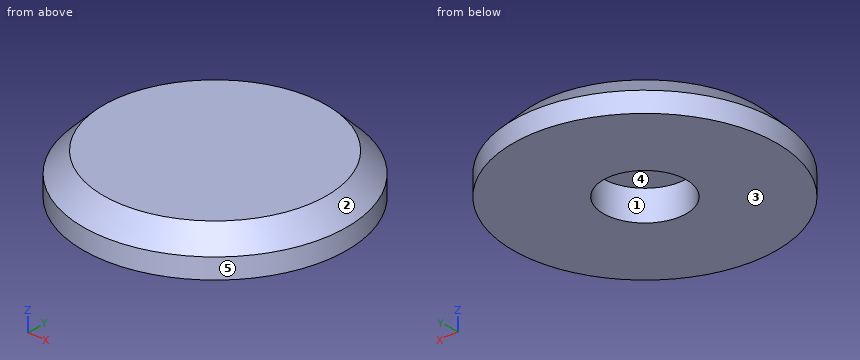
```python
from build123d import *

# Parameters (mm, degrees)
SKETCH1_R           = 3.7
BOSS_EXTRUDE1_DEPTH = 10
SKETCH2_R           = 5
BOSS_EXTRUDE2_DEPTH = 2
SKETCH3_R           = 13
SKETCH3_R_2         = 4.1
BOSS_EXTRUDE3_DEPTH = 4
SKETCH4_R           = 21.887313971
CUT_EXTRUDE1_DEPTH  = 23
CHAMFER2_SIZE       = 2
SKETCH5_R           = 5.500381587
BOSS_EXTRUDE4_DEPTH = 1


with BuildPart() as part:
    # Sketch1 → Boss-Extrude1 (new body)
    with BuildSketch(Plane.XY):
        Circle(SKETCH1_R)
    extrude(amount=BOSS_EXTRUDE1_DEPTH)

    # Sketch2 → Boss-Extrude2 (add)
    with BuildSketch(Plane(origin=(0, 0, 0), x_dir=(-1, 0, 0), z_dir=(0, 0, -1))):
        Circle(SKETCH2_R)
    extrude(amount=BOSS_EXTRUDE2_DEPTH)

    # Sketch4 → Cut-Extrude1 (cut)
    with BuildSketch(Plane(origin=(0, 0, 10), x_dir=(-1, 0, 0), z_dir=(0, 0, -1))):
        with Locations((0, 0.481738505)):
            Circle(SKETCH4_R)
    extrude(amount=CUT_EXTRUDE1_DEPTH, mode=Mode.SUBTRACT)


with BuildPart() as body_2:
    # Sketch3 → Boss-Extrude3 (new body)
    with BuildSketch(Plane.XY.offset(10)):
        Circle(SKETCH3_R)
        Circle(SKETCH3_R_2, mode=Mode.SUBTRACT)
    extrude(amount=BOSS_EXTRUDE3_DEPTH)

    # Chamfer2
    chamfer2_edges = [body_2.edges().sort_by_distance(p)[0] for p in [
        (-13, 0, 14),
    ]]
    chamfer(chamfer2_edges, length=CHAMFER2_SIZE)

    # Sketch5 → Boss-Extrude4 (add)
    with BuildSketch(Plane.XY.offset(14)):
        Circle(SKETCH5_R)
    extrude(amount=-BOSS_EXTRUDE4_DEPTH)


solid = body_2.part
```
Input: part model. Units: mm. Frame: model coordinates. Face numbers are marked on the shaded views. A direction names the side the tool comes from. Give positions to 0.01 mm unless a question says otherwise; leave off trailing zeros. Write each loop counter-clockwise with the first axis right and the second up, starting at its lowest first coordinate (ties: lowest second). Pieces come first, ordered by that corner, then holes. Notation, with made-up numbers: (-7.75, 19) - (49.25, 19) arc R23 ccw to (49.25, 39) - close; hole circle Ø2 at (82.5, -34.5). An arc over 180 degrees is marked (long way). Write item = value, one per line. Start each with the question number.
1. Section query C-C, the plane z = 11.15. Output: boundary loops of the cut face in (x, y).
2. Access query for the marked faces 4 and 5. Directions: +Z, -Z, +X, -X, +Y, -Y. A direction counts if a zero-diameter tool reaches every point of the face in a straight line with its end or side. Return the directions, or none.
3. Mould query, pull axis Y, two halves, no side actions, for the marked faces 1, 2 and 3. Classes: released by +Y, released by -Y, zero draft, split by the parting line, or undercut.
4. First-contact query: pin 1 Ø1.5 at (y, z) = (4, 12) entering from -X; pin 2 Ø1.5 at (x, z) = (-2, 12.5) entering from +Y; pin 3 Ø4 at (x, y) = (-0.5, 2) entering from -Z. Flat tips, straight axial feed; report the tip coordinate or a pass-through.
5. Section query A-A, the plane y = 0. Output: boundary loops of the cut face in (x, z).
6. Ray query, L1, parallel to Y at x = 0, z = 10.9; L2, parallel to Y at x = 1, z = 12.35; L3, parallel to X at y = -2.5, z = 12.1. Return the intervals inside material, ascending.
Check sheet entries:
q1.outline = circle Ø26 at (0, 0); hole circle Ø8.2 at (0, 0)
q2.face_4 = -Z
q2.face_5 = +Z, -Z
q3.face_1 = undercut
q3.face_2 = split by the parting line
q3.face_3 = zero draft
q4.pin_1 = -12.59
q4.pin_2 = 12.92
q4.pin_3 = 13
q5.outline = (-13, 10) - (-4.1, 10) - (-4.1, 13) - (4.1, 13) - (4.1, 10) - (13, 10) - (13, 12) - (11, 14) - (-11, 14) - (-13, 12) - close
q6.L1 = -13 to -4.1, 4.1 to 13
q6.L2 = -12.61 to -3.98, 3.98 to 12.61
q6.L3 = -12.66 to -3.25, 3.25 to 12.66
